The model under review builds one solid part; all positions refer to its coordinate system, in mm. A direction names the side the tool comes from. Give positions to 0.01 mm unless a question says otherwise; leave off trailing zeros. Order: outer loops, then holes, each group sorted by start corner. A loop starts at its lowest first (then second) coordinate and runs counter-clockwise, first axis right, second up.
```python
from build123d import *

# Parameters (mm, degrees)
SKETCH_1_W          = 20
SKETCH_1_H          = 5
EXTRUDE_1_DEPTH     = 15
FILLET_1_R          = 3
SKETCH_3_R          = 2.6
CUT_EXTRUDE_1_DEPTH = 50.523353077
SKETCH_9_R          = 4.5
SKETCH_9_R_2        = 3.5
CUT_EXTRUDE_2_DEPTH = 2
FILLET_2_R          = 1


with BuildPart() as part:
    # 草图1 → 凸台-拉伸1 (new body)
    with BuildSketch(Plane.XY):
        Polygon((-10, 27.75), (-20, 0), (0, 0), (0, 42.75), (-10, 42.75), align=None)
        with Locations((-10, -2.5)):
            Rectangle(SKETCH_1_W, SKETCH_1_H)
    extrude(amount=EXTRUDE_1_DEPTH)

    # 圆角1
    fillet_1_edges = [part.edges().sort_by_distance(p)[0] for p in [
        (-5, 42.75, 15),
        (-5, 42.75, 0),
    ]]
    fillet(fillet_1_edges, radius=FILLET_1_R)

    # 草图3 → 切除-拉伸1 (cut, through all)
    with BuildSketch(Plane(origin=(0, 0, 0), x_dir=(0, 0, -1), z_dir=(1, 0, 0))):
        with Locations((-7.5, 35.25)):
            Circle(SKETCH_3_R)
    extrude(amount=-CUT_EXTRUDE_1_DEPTH, mode=Mode.SUBTRACT)

    # 草图9 → 切除-拉伸2 (cut)
    with BuildSketch(Plane.ZY.offset(10)):
        with Locations(Location((7.5, 35.25, 0), (0, 0, 270))):
            Circle(SKETCH_9_R)
        with Locations(Location((7.5, 35.25, 0), (0, 0, 270))):
            Circle(SKETCH_9_R_2, mode=Mode.SUBTRACT)
    extrude(amount=-CUT_EXTRUDE_2_DEPTH, mode=Mode.SUBTRACT)

    # 圆角2
    # the kernel refuses this fillet: 1 mm, written as the material it takes off along each edge
    with BuildSketch(Plane(origin=(-10, 35.25, 7.5), x_dir=(0, 0, -1), z_dir=(0, -1, 0))) as fillet_2_piece_1:
        with BuildLine():
            CenterArc((3.6, 0.994987437), FILLET_2_R, 180, 84.260829523)
            Line((3.5, 0), (3.498, -0.019899749))
            ThreePointArc((3.498, -0.019899749), (3.05, -0.02), (2.6, -0.02))
            Line((2.6, -0.02), (2.58, 0))
            Line((2.58, 0), (2.58, 0.994987437))
            Line((2.58, 0.994987437), (2.6, 0.994987437))
        make_face()
    revolve(axis=Axis((-10, 35.25, 7.5), (1, 0, 0)), mode=Mode.SUBTRACT)


solid = part.part
```
Item 1: Take a section at B-B (y = 35.25). Give the boundary of the cut face in (x, z), and give its area (3 significant figures).
Values found:
outline: (-10, 0) - (0, 0) - (0, 4.9) - (-9.01, 4.9) arc R1 ccw to (-10, 4) - (-8, 4) - (-8, 3) - (-10, 3) - close; (-10, 11) arc R1 ccw to (-9.01, 10.1) - (0, 10.1) - (0, 15) - (-10, 15) - (-10, 12) - (-8, 12) - (-8, 11) - close
area: 93.6 mm2
Item 2: Take a section at A-A (z = 7.5). Give the boundary of the cut face in (x, y).
Values found:
outline: (-20, -5) - (0, -5) - (0, 32.65) - (-9.01, 32.65) arc R1 ccw to (-10, 31.75) - (-8, 31.75) - (-8, 30.75) - (-10, 30.75) - (-10, 27.75) - (-20, 0) - close; (-10, 38.75) arc R1 ccw to (-9.01, 37.85) - (0, 37.85) - (0, 42.75) - (-10, 42.75) - (-10, 39.75) - (-8, 39.75) - (-8, 38.75) - close
Item 3: Take a section at C-C (x = -7.5). Give the boundary of the cut face in (y, z), and give its area (3 significant figures).
Values found:
outline: (-5, 0) - (39.75, 0) arc R3 ccw to (42.75, 3) - (42.75, 12) arc R3 ccw to (39.75, 15) - (-5, 15) - close; hole circle Ø5.2 at (35.25, 7.5)
area: 691 mm2
Item 4: Clearance check with flat-ended pins moving along their axes: pin 1 Ø7 at (y, z) = (35.25, 7.5) entering from -X; pin 2 Ø6 at (y, z) = (8, 10) entering from -X; pin 3 Ø3 at (y, z) = (19.5, 1.5) entering from +X; pin 4 Ø1 at (y, z) = (27, 13) entering from -X. State where each tip first meets the part, or that it passes through.
Values found:
pin 1: stops at x = -10
pin 2: stops at x = -18.2
pin 3: stops at x = 0
pin 4: stops at x = -10.45
Item 5: Take a section at D-D (x = -9.5). Give the boundary of the cut face in (y, z), and give its area (3 significant figures).
Values found:
outline: (-5, 0) - (39.75, 0) arc R3 ccw to (42.75, 3) - (42.75, 12) arc R3 ccw to (39.75, 15) - (-5, 15) - close; circle Ø7 at (35.25, 7.5); hole circle Ø9 at (35.25, 7.5); hole circle Ø5.46 at (35.25, 7.5)
area: 664 mm2
Item 6: For line 1 (Y direction, x = -3.75, z = 7.5); line 2 (X direction, y = 28, z = 6.25); line 3 (X direction, y = 6.5, z = 2.25), list the stretches that pass through material, from the lowest coordinate up.
Values found:
line 1: y = -5 to 32.65, 37.85 to 42.75
line 2: x = -10 to 0
line 3: x = -17.66 to 0
Item 7: For faces 1 (the flat face through (-8, 13, 0)), 2 (the flat face through (-10, 32, 11)), 3 (the flat face through (-8, 38, 5)), list the 3-axis set-ups (+Z, -Z, +X, -X, +Y, -Y) from which the entire face can be reached by the end or side of a thin tool; tool diameter is ignored.
Values found:
face 1: -Z, +X, -X, +Y, -Y
face 2: +Z, -Z, -X, +Y
face 3: -X
